The listing builds one solid part. Answer for the finished solid, in the listing's coordinates (mm). A direction names the side the tool comes from. Give positions to 0.01 mm unless a question says otherwise; leave off trailing zeros. Write each loop counter-clockwise with the first axis right and the second up, starting at its lowest first coordinate (ties: lowest second). Pieces come first, ordered by that corner, then holes. Notation, with made-up numbers: (-12.75, -17) -> (29.25, -17) arc R7 ccw to (29.25, -6) -> close; hole circle Ø1 at (32, 78.25). An arc over 180 degrees is marked (long way). Use CSV: the item, a comma, the result in double quotes. Start each with the question number.
from build123d import *

# Parameters (mm, degrees)
F0_R     = 4.4487015319
F0_R_2   = 10.7530048188
F0_R_3   = 4.7180127793
F1_DEPTH = 25.4


with BuildPart() as f1:
    # F0 (on Front) → F1 (new body)
    with BuildSketch(Plane.XZ):
        with BuildLine():
            ThreePointArc((-29.4424401282, 3.4015260978), (-23.0262753535, 9.9406396762), (-16.1905688202, 16.0398439684))
            ThreePointArc((-16.1905688202, 16.0398439684), (-14.9730955589, 25.3716641264), (-13.2094991853, 34.6158426424))
            ThreePointArc((-13.2094991853, 34.6158426424), (-33.2950660075, 42.3616642817), (-54.3334142599, 46.9240814309))
            ThreePointArc((-54.3334142599, 46.9240814309), (-43.9313490235, 23.9941508784), (-29.4424401282, 3.4015260978))
        make_face()
        with BuildLine():
            ThreePointArc((-0.2127594199, 27.5427215846), (6.3768354794, 31.3598309723), (13.1668725149, 34.8077987896))
            ThreePointArc((13.1668725149, 34.8077987896), (7.721142089, 53.7045907434), (0, 71.7912900237))
            ThreePointArc((0, 71.7912900237), (-7.7540886954, 53.6119593723), (-13.2094991853, 34.6158426424))
            ThreePointArc((-13.2094991853, 34.6158426424), (-6.6172580099, 31.2517690189), (-0.2127594199, 27.5427215846))
        make_face()
        with Locations((0, 49.6207140386)):
            Circle(F0_R, mode=Mode.SUBTRACT)
        with BuildLine():
            ThreePointArc((13.1668725149, 34.8077987896), (14.9841600378, 25.3026214649), (16.223923099, 15.7050218969))
            ThreePointArc((16.223923099, 15.7050218969), (22.9196518716, 9.724571518), (29.2167284259, 3.3257124477))
            ThreePointArc((29.2167284259, 3.3257124477), (43.8176697051, 23.9481716961), (54.3334142599, 46.9240814309))
            ThreePointArc((54.3334142599, 46.9240814309), (33.2765171586, 42.4751427427), (13.1668725149, 34.8077987896))
        make_face()
        with BuildLine():
            ThreePointArc((-0.1224819877, -22.2551113905), (8.5491454913, -16.1687348266), (16.7184581773, -9.4231115752))
            ThreePointArc((16.7184581773, -9.4231115752), (16.9649715432, 3.1506730326), (16.223923099, 15.7050218969))
            ThreePointArc((16.223923099, 15.7050218969), (8.2207799897, 21.9226750358), (-0.2127594199, 27.5427215846))
            ThreePointArc((-0.2127594199, 27.5427215846), (-8.4069648764, 22.0764511026), (-16.1905688202, 16.0398439684))
            ThreePointArc((-16.1905688202, 16.0398439684), (-16.9635494943, 3.2221192601), (-16.7069505399, -9.6163277953))
            ThreePointArc((-16.7069505399, -9.6163277953), (-8.6597139653, -16.2572027994), (-0.1224819877, -22.2551113905))
        make_face()
        Circle(F0_R_2, mode=Mode.SUBTRACT)
        with BuildLine():
            ThreePointArc((-13.2094991853, 34.6158426424), (-14.9730955589, 25.3716641264), (-16.1905688202, 16.0398439684))
            ThreePointArc((-16.1905688202, 16.0398439684), (-8.4069648764, 22.0764511026), (-0.2127594199, 27.5427215846))
            ThreePointArc((-0.2127594199, 27.5427215846), (-6.6172580099, 31.2517690189), (-13.2094991853, 34.6158426424))
        make_face()
        with BuildLine():
            ThreePointArc((-0.2127594199, 27.5427215846), (8.2207799897, 21.9226750358), (16.223923099, 15.7050218969))
            ThreePointArc((16.223923099, 15.7050218969), (14.9841600378, 25.3026214649), (13.1668725149, 34.8077987896))
            ThreePointArc((13.1668725149, 34.8077987896), (6.3768354794, 31.3598309723), (-0.2127594199, 27.5427215846))
        make_face()
        with BuildLine():
            ThreePointArc((-57.542737113, -42.9281111723), (-35.2995419272, -38.3673220516), (-14.1309868657, -30.1543563216))
            ThreePointArc((-14.1309868657, -30.1543563216), (-15.7511847912, -19.9270099612), (-16.7069505399, -9.6163277953))
            ThreePointArc((-16.7069505399, -9.6163277953), (-23.2950130239, -3.3229397285), (-29.4424401282, 3.4015260978))
            ThreePointArc((-29.4424401282, 3.4015260978), (-45.7877840818, -18.3711885214), (-57.542737113, -42.9281111723))
        make_face()
        with BuildLine():
            ThreePointArc((-29.4424401282, 3.4015260978), (-23.2950130239, -3.3229397285), (-16.7069505399, -9.6163277953))
            ThreePointArc((-16.7069505399, -9.6163277953), (-16.9635494943, 3.2221192601), (-16.1905688202, 16.0398439684))
            ThreePointArc((-16.1905688202, 16.0398439684), (-23.0262753535, 9.9406396762), (-29.4424401282, 3.4015260978))
        make_face()
        with BuildLine():
            ThreePointArc((-16.7069505399, -9.6163277953), (-15.7511847912, -19.9270099612), (-14.1309868657, -30.1543563216))
            ThreePointArc((-14.1309868657, -30.1543563216), (-7.0093726235, -26.4128630389), (-0.1224819877, -22.2551113905))
            ThreePointArc((-0.1224819877, -22.2551113905), (-8.6597139653, -16.2572027994), (-16.7069505399, -9.6163277953))
        make_face()
        with BuildLine():
            ThreePointArc((-14.1309868657, -30.1543563216), (-8.5014831961, -51.4601778042), (0, -71.7912900237))
            ThreePointArc((0, -71.7912900237), (8.482288282, -51.5167009706), (14.1084600409, -30.2715987794))
            ThreePointArc((14.1084600409, -30.2715987794), (6.8713335487, -26.4793190065), (-0.1224819877, -22.2551113905))
            ThreePointArc((-0.1224819877, -22.2551113905), (-7.0093726235, -26.4128630389), (-14.1309868657, -30.1543563216))
        make_face()
        with Locations((0, -51.7978556454)):
            Circle(F0_R_3, mode=Mode.SUBTRACT)
        with BuildLine():
            ThreePointArc((16.7184581773, -9.4231115752), (15.7557958243, -19.8902119169), (14.1084600409, -30.2715987794))
            ThreePointArc((14.1084600409, -30.2715987794), (35.2902850673, -38.4369294065), (57.542737113, -42.9281111723))
            ThreePointArc((57.542737113, -42.9281111723), (45.6499453561, -18.4109129726), (29.2167284259, 3.3257124477))
            ThreePointArc((29.2167284259, 3.3257124477), (23.1779099268, -3.2548828175), (16.7184581773, -9.4231115752))
        make_face()
        with BuildLine():
            ThreePointArc((16.223923099, 15.7050218969), (16.9649715432, 3.1506730326), (16.7184581773, -9.4231115752))
            ThreePointArc((16.7184581773, -9.4231115752), (23.1779099268, -3.2548828175), (29.2167284259, 3.3257124477))
            ThreePointArc((29.2167284259, 3.3257124477), (22.9196518716, 9.724571518), (16.223923099, 15.7050218969))
        make_face()
        with BuildLine():
            ThreePointArc((-0.1224819877, -22.2551113905), (6.8713335487, -26.4793190065), (14.1084600409, -30.2715987794))
            ThreePointArc((14.1084600409, -30.2715987794), (15.7557958243, -19.8902119169), (16.7184581773, -9.4231115752))
            ThreePointArc((16.7184581773, -9.4231115752), (8.5491454913, -16.1687348266), (-0.1224819877, -22.2551113905))
        make_face()
    extrude(amount=F1_DEPTH)


solid = f1.part
Q1. Section C-C on y = -15.25 is taken. Give the vertices of the cut face in (x, z).
Q2. Straight lines are drawn through the part: L1, parallel to Z at x = -4, y = -16.5; L2, parallel to Z at x = -1.5, y = -10.5; L3, parallel to X at y = -17, z = -34. For each, find the intervals that lie inside material, in ascending order.
Q3. Section B-B on x = -39 is taken. Give the vertices of the cut face in (y, z), then the cut area to 3 significant figures.
Q4. Section A-A on z = 0 is taken. Give the vertices of the cut face in (x, y), then the cut area to 3 significant figures.
Q5. The mould has two halves that part along Z. Classify faces 1 (the face through (-44.106, -12.522, 24.301)), 2 (the face through (-8.6, -12.52, -51.17)), 3 (the face through (33.57, -12.52, 42.56)): +Z half, -Z half, draft (parallel to the pull), parting line (faces both ways), or undercut.
Q6. Section D-D on x = -22.5 is taken. Give the vertices of the cut face in (y, z), then the cut area to 3 significant figures.
Q7. Flat-ended cylindrical pins translate along their axes: pin 1 Ø12 at (y, z) = (-12, 15.5) entering from -X; pin 2 Ø5.5 at (x, z) = (0, -51.8) entering from +Y; pin 3 Ø2 at (x, z) = (28.5, 31.5) entering from +Y; pin 4 Ø4 at (y, z) = (-22, -5) entering from +X. Find the tip coordinate at first contact, or state that the pin passes through.
Q8. For faces 4 (the face through (-35.605, -12.522, -38.457)), 5 (the face through (-33.006, -12.522, 42.275)), 6 (the face through (45.85, -12.52, -18.74)), 7 (the face through (-45.589, -12.522, -18.045)), determine the directions among +Z, -Z, +X, -X, +Y, -Y from which every point of the face is accessible in a straight line to the end or side of a thin tool.
Output:
1,outline,"(-57.54, -42.93) arc R135.42 ccw to (-14.13, -30.15) arc R160.12 ccw to (0, -71.79) arc R160.12 ccw to (14.11, -30.27) arc R134.66 ccw to (57.54, -42.93) arc R139.46 ccw to (29.22, 3.33) arc R135.42 ccw to (54.33, 46.92) arc R138.06 ccw to (13.17, 34.81) arc R160.12 ccw to (0, 71.79) arc R160.12 ccw to (-13.21, 34.62) arc R139.46 ccw to (-54.33, 46.92) arc R134.66 ccw to (-29.44, 3.4) arc R138.06 ccw to start; hole circle Ø21.51 at (0, 0); hole circle Ø9.44 at (0, -51.8); hole circle Ø8.9 at (0, 49.62)"
2,L1,"-63.19 to -54.3, -49.3 to -9.98, 9.98 to 47.67, 51.57 to 63.19"
2,L2,"-68.72 to -56.27, -47.32 to -10.65, 10.65 to 45.43, 53.81 to 68.72"
2,L3,"-53.95 to -22.76, -13.34 to 13.34, 22.5 to 53.89"
3,outline,"(-25.4, -39.4) -> (0, -39.4) -> (0, -8.22) -> (-25.4, -8.22) -> close; (-25.4, 16.03) -> (0, 16.03) -> (0, 43.94) -> (-25.4, 43.94) -> close"
3,area,"1,500 mm²"
4,outline,"(-32.46, -25.4) -> (-10.75, -25.4) -> (-10.75, 0) -> (-32.46, 0) -> close; (10.75, -25.4) -> (32.19, -25.4) -> (32.19, 0) -> (10.75, 0) -> close"
4,area,"1,100 mm²"
5,face 1,"undercut"
5,face 2,"-Z half"
5,face 3,"+Z half"
6,outline,"(-25.4, -33.89) -> (0, -33.89) -> (0, 38.64) -> (-25.4, 38.64) -> close"
6,area,"1,840 mm²"
7,pin 1,"x = -42.47"
7,pin 2,"through"
7,pin 3,"y = 0"
7,pin 4,"x = 37.86"
8,face 4,"-Z, +Y, -Y"
8,face 5,"+Z, +Y, -Y"
8,face 6,"+X, +Y, -Y"
8,face 7,"-X, +Y, -Y"
